```python
from build123d import *

# Parameters (mm, degrees)
F0_W      = 10
F0_H      = 60
F1_DEPTH  = 55
F2_W      = 220
F2_H      = 110
F3_DEPTH  = 10
F5_R      = 10
F6_DEPTH  = 10
F7_R      = 5
F8_DEPTH  = 10
F9_R      = 5
F9_R_2    = 6
F10_DEPTH = 3
F11_R     = 6
F12_DEPTH = 60.001


with BuildPart() as f1:
    # F0 (on Right) → F1 (new body, symmetric)
    with BuildSketch(Plane.YZ):
        Polygon((100, 10), (100, 0), (100, -40), (110, -40), (110, 70), (100, 70), align=None)
        Polygon((50, 10), (-100, 10), (-100, 0), (100, 0), (100, 10), (60, 10), align=None)
        with Locations((55, 40)):
            Rectangle(F0_W, F0_H)
        Polygon((-100, 70), (-110, 70), (-110, -40), (-100, -40), (-100, 0), (-100, 10), align=None)
    extrude(amount=F1_DEPTH, both=True)

    # F2 (on face) → F3 (join)
    with BuildSketch(Plane.YZ.offset(55)):
        with Locations((0, 15)):
            Rectangle(F2_W, F2_H)
    extrude(amount=F3_DEPTH)

    # F4: F1 across plane


with BuildPart() as f1_1:
    add(f1.part)
    add(f1.part.mirror(Plane.YZ))

    # F5 (on face) → F6 (cut, through all)
    with BuildSketch(Plane(origin=(0, 110, 0), x_dir=(-1, 0, 0), z_dir=(0, 1, 0))):
        with Locations((0, 40)):
            Circle(F5_R)
    extrude(amount=-F6_DEPTH, mode=Mode.SUBTRACT)

    # F7 (on face) → F8 (cut, through all)
    with BuildSketch(Plane.XZ.offset(-50)):
        with Locations((0, 40)):
            Circle(F7_R)
    extrude(amount=-F8_DEPTH, mode=Mode.SUBTRACT)

    # F9 (on face) → F10 (cut)
    with BuildSketch(Plane(origin=(0, -100, 0), x_dir=(-1, 0, 0), z_dir=(0, 1, 0))):
        with Locations((0, 40)):
            Circle(F9_R)
        with Locations((35, 40)):
            Circle(F9_R_2)
        with Locations((-35, 40)):
            Circle(F9_R_2)
    extrude(amount=-F10_DEPTH, mode=Mode.SUBTRACT)

    # F11 (on face) → F12 (cut, through all)
    with BuildSketch(Plane.XZ.offset(-50)):
        with Locations((-35, 40)):
            Circle(F11_R)
        with Locations((35, 40)):
            Circle(F11_R)
    extrude(amount=-F12_DEPTH, mode=Mode.SUBTRACT)


solid = f1_1.part
```
Verification items for the finished model (mm, model axes). A direction names the side the tool comes from. Coordinates: 2 decimals unless noted, no trailing zeros. Order: outer loops, then holes, each group sorted by start corner. A loop starts at its lowest first (then second) coordinate and runs counter-clockwise, first axis right, second up. Notation, with made-up numbers: (86.5, -11.5) -> (113.5, -11.5) arc R30 cw to (113.5, 10.5) -> close; hole circle Ø1 at (-34.5, 83.5). An arc over 180 degrees is marked (long way). Answer as CSV lines item,"result". Start each with the question number.
1) Set-up check for faces 4 (the face through (39.76, -101.48, 36.35)), 5 (the face through (55, -1, -20)), 6 (the face through (-65, -2, 16)), 7 (the face through (1, 110, 14)), 8 (the face through (1, -100, 46)): record each of +Z, -Z, +X, -X, +Y, -Y from which the full face is reachable in a straight line by a thin tool's end or side.
2) Cross-section at A-A, the plane x = 0. Record the boundary of the cut face in (y, z).
3) Release check for a two-part mould opening along Z. For faces 1 (the face through (0, -103, 40)), 2 (the face through (-57, -9, -40)), 3 (the face through (-55, -26, 40)) record: released by +Z, released by -Z, zero draft, split by the parting line, or undercut.
4) Cross-section at D-D, the plane x = -15. Record the boundary of the cut face in (y, z).
5) Gauge pin test, flat ends, axial feed: pin 1 Ø12 at (x, y) = (29, 74) entering from +Z; pin 2 Ø11 at (x, z) = (-35, 40) entering from +Y. Record the tip position at first contact, or that the pin passes through.
6) Material ranges on L1, parallel to Y at x = 30, z = 48.5; L2, parallel to X at y = 10, z = 53.5; L3, parallel to Z at x = 0, y = -100.95, recorded low to high. Write a range as [from, to].
7) Cross-section at B-B, the plane z = -24.5. Record the boundary of the cut face in (x, y), then the cut area to 3 significant figures.
8) Cross-section at C-C, the plane z = 52.5. Record the boundary of the cut face in (x, y), then the cut area to 3 significant figures.
Conclusion:
1,face 4,"+Y"
1,face 5,"-Z"
1,face 6,"+Z, -Z, -X, +Y, -Y"
1,face 7,"+Z, -Z, +X, -X, +Y"
1,face 8,"+Z"
2,outline,"(-110, -40) -> (-100, -40) -> (-100, 0) -> (100, 0) -> (100, -40) -> (110, -40) -> (110, 30) -> (100, 30) -> (100, 10) -> (60, 10) -> (60, 35) -> (50, 35) -> (50, 10) -> (-100, 10) -> (-100, 35) -> (-103, 35) -> (-103, 45) -> (-100, 45) -> (-100, 70) -> (-110, 70) -> close; (50, 45) -> (60, 45) -> (60, 70) -> (50, 70) -> close; (100, 50) -> (110, 50) -> (110, 70) -> (100, 70) -> close"
3,face 1,"undercut"
3,face 2,"released by -Z"
3,face 3,"zero draft"
4,outline,"(-110, -40) -> (-100, -40) -> (-100, 0) -> (100, 0) -> (100, -40) -> (110, -40) -> (110, 70) -> (100, 70) -> (100, 10) -> (60, 10) -> (60, 70) -> (50, 70) -> (50, 10) -> (-100, 10) -> (-100, 70) -> (-110, 70) -> close"
5,pin 1,"stops at z = 10"
5,pin 2,"stops at y = -103"
6,L1,"y = [-110, -100], [50, 60], [100, 110]"
6,L2,"x = [-65, -55], [55, 65]"
6,L3,"z = [-40, 35], [45, 70]"
7,outline,"(-65, -110) -> (65, -110) -> (65, 110) -> (-65, 110) -> close; hole (-55, -100) -> (55, -100) -> (55, 100) -> (-55, 100) -> close"
7,area,"6,600 mm²"
8,outline,"(-65, -110) -> (65, -110) -> (65, 110) -> (-65, 110) -> close; hole (-55, -100) -> (55, -100) -> (55, 50) -> (-55, 50) -> close; hole (-55, 60) -> (55, 60) -> (55, 100) -> (-55, 100) -> close"
8,area,"7,700 mm²"
